from build123d import *

# Parameters (mm, degrees)
SKETCH1_W               = 120
SKETCH1_H               = 24
BOSS_EXTRUDE1_DEPTH     = 3
SKETCH2_W               = 10
SKETCH2_H               = 3
CUT_EXTRUDE1_DEPTH      = 4
MIRROR3_COPY_1_SKETCH_W = 10
MIRROR3_COPY_1_SKETCH_H = 3
MIRROR3_COPY_1_DEPTH    = 4
SKETCH3_W               = 3
SKETCH3_H               = 8
SKETCH3_H_2             = 10
CUT_EXTRUDE2_DEPTH      = 4


with BuildPart() as part:
    # Sketch1 → Boss-Extrude1 (new body)
    with BuildSketch(Plane.XY):
        Rectangle(SKETCH1_W, SKETCH1_H)
    extrude(amount=BOSS_EXTRUDE1_DEPTH)

    # Sketch2 → Cut-Extrude1 (cut, through all)
    with BuildSketch(Plane.XY.offset(3)):
        with Locations((15, 10.5)):
            Rectangle(SKETCH2_W, SKETCH2_H)
        with Locations((35, 10.5)):
            Rectangle(SKETCH2_W, SKETCH2_H)
        with Locations((55, 10.5)):
            Rectangle(SKETCH2_W, SKETCH2_H)
    cut_extrude1 = extrude(amount=-CUT_EXTRUDE1_DEPTH, mode=Mode.SUBTRACT)

    # Mirror2: Cut-Extrude1 across plane
    add(cut_extrude1.mirror(Plane(origin=(0, 0, 0), x_dir=(0, 0, 1), z_dir=(1, 0, 0))), mode=Mode.SUBTRACT)

    # Mirror3: Cut-Extrude1 across plane
    add(cut_extrude1.mirror(Plane.ZX), mode=Mode.SUBTRACT)

    # Mirror3 copy 1 sketch → Mirror3 copy 1 (cut, through all)
    with BuildSketch(Plane(origin=(0, 0, 3), x_dir=(-1, 0, 0), z_dir=(0, 0, 1))):
        with Locations((15, 10.5)):
            Rectangle(MIRROR3_COPY_1_SKETCH_W, MIRROR3_COPY_1_SKETCH_H)
        with Locations((35, 10.5)):
            Rectangle(MIRROR3_COPY_1_SKETCH_W, MIRROR3_COPY_1_SKETCH_H)
        with Locations((55, 10.5)):
            Rectangle(MIRROR3_COPY_1_SKETCH_W, MIRROR3_COPY_1_SKETCH_H)
    extrude(amount=-MIRROR3_COPY_1_DEPTH, mode=Mode.SUBTRACT)

    # Sketch3 → Cut-Extrude2 (cut, through all)
    with BuildSketch(Plane.XY.offset(3)):
        with Locations((24, 0)):
            Rectangle(SKETCH3_W, SKETCH3_H)
        with Locations((-24, 0)):
            Rectangle(SKETCH3_W, SKETCH3_H)
        with Locations((58.5, 0)):
            Rectangle(SKETCH3_W, SKETCH3_H_2)
        with Locations((-58.5, 0)):
            Rectangle(SKETCH3_W, SKETCH3_H_2)
    extrude(amount=-CUT_EXTRUDE2_DEPTH, mode=Mode.SUBTRACT)


solid = part.part
Read the model definition and answer for the solid it produces. Units are mm, in the model's axes. A direction names the side the tool comes from. Round coordinates to 2 decimals unless told otherwise and drop trailing zeros. Write each loop counter-clockwise with the first axis right and the second up, starting at its lowest first coordinate (ties: lowest second). Pieces come first, ordered by that corner, then holes. Notation, with made-up numbers: (50.25, 81) - (54.25, 81) arc R19 ccw to (54.25, 91) - close; hole circle Ø2 at (-35.75, 14.25). An arc over 180 degrees is marked (long way). Use a Markdown table: item, result.
(1) The mould has two halves that part along Y. Classify faces 5 (the flat face through (-59, -5, 2)), 6 (the flat face through (-40, -10, 2)), 7 (the flat face through (-15, -9, 2)): released by +Y, released by -Y, zero draft, split by the parting line, or undercut.
Reported:
| item | result |
|---|---|
| face 5 | undercut |
| face 6 | zero draft |
| face 7 | released by -Y |
(2) The part is cut by section C-C (z = 1.7). State how many separate pieces and enclosed holes the cut face has, then the cut area to 3 significant figures.
Reported:
| item | result |
|---|---|
| separate pieces | 1 |
| enclosed holes | 2 |
| area | 2,410 mm2 |
(3) Each of these flat-tipped pins is pushed along its axis until it touches: pin 1 Ø0.9 at (x, z) = (-58, 1.5) entering from +Y; pin 2 Ø1.5 at (y, z) = (10.5, 1.5) entering from +X; pin 3 Ø0.9 at (y, z) = (1, 2) entering from -X. Where does it stop, or does it pass through?
Reported:
| item | result |
|---|---|
| pin 1 | y = 9 |
| pin 2 | x = 50 |
| pin 3 | x = -57 |
(4) The part is cut by section D-D (x = 38.5). Write down the section's boundary in (y, z).
Reported:
| item | result |
|---|---|
| outline | (-9, 0) - (9, 0) - (9, 3) - (-9, 3) - close |
(5) The part is cut by section A-A (y = -10.25). Write down the section's boundary in (x, z), then the cut area to 3 significant figures.
Reported:
| item | result |
|---|---|
| outline | (-50, 0) - (-40, 0) - (-40, 3) - (-50, 3) - close; (-30, 0) - (-20, 0) - (-20, 3) - (-30, 3) - close; (-10, 0) - (10, 0) - (10, 3) - (-10, 3) - close; (20, 0) - (30, 0) - (30, 3) - (20, 3) - close; (40, 0) - (50, 0) - (50, 3) - (40, 3) - close |
| area | 180 mm2 |
(6) Straight lines are drawn through the part: line 1 along X through (y, z) = (-10.25, 0.3); line 2 along X through (y, z) = (-0.5, 1.75); line 3 along X through (y, z) = (4.75, 0.25). For each, find the intervals that lie inside material, in ascending order. Write a range as [from, to].
Reported:
| item | result |
|---|---|
| line 1 | [-50, -40], [-30, -20], [-10, 10], [20, 30], [40, 50] |
| line 2 | [-57, -25.5], [-22.5, 22.5], [25.5, 57] |
| line 3 | [-57, 57] |
(7) Which of the six approach directions +Z, -Z, +X, -X, +Y, -Y give full straight-line access (tool end or side, diameter ignored) to faces 1 (the flat face through (-24, 4, 2)), 2 (the flat face through (50, -10, 2)), 3 (the flat face through (58, 5, 2)), 4 (the flat face through (-35, -9, 2))?
Reported:
| item | result |
|---|---|
| face 1 | +Z, -Z |
| face 2 | +Z, -Z, +X, -Y |
| face 3 | +Z, -Z, +X |
| face 4 | +Z, -Z, -Y |
(8) The part is cut by section B-B (y = -0.25). Write down the section's boundary in (x, z).
Reported:
| item | result |
|---|---|
| outline | (-57, 0) - (-25.5, 0) - (-25.5, 3) - (-57, 3) - close; (-22.5, 0) - (22.5, 0) - (22.5, 3) - (-22.5, 3) - close; (25.5, 0) - (57, 0) - (57, 3) - (25.5, 3) - close |
